The drawing under review shows one solid part. Ordinate dimensions are in mm from its lowest x, y, z. Coordinates: 2 decimals unless noted, no trailing zeros. Order: outer loops, then holes, each group sorted by start corner. A loop starts at its lowest first (then second) coordinate and runs counter-clockwise, first axis right, second up. Notation, with made-up numbers: (3.25, 6) - (51.25, 6) arc R9 ccw to (51.25, 21) - close; hole circle Ø6 at (-39.75, 51). An arc over 180 degrees is marked (long way). Answer in a Markdown table with one row per item.
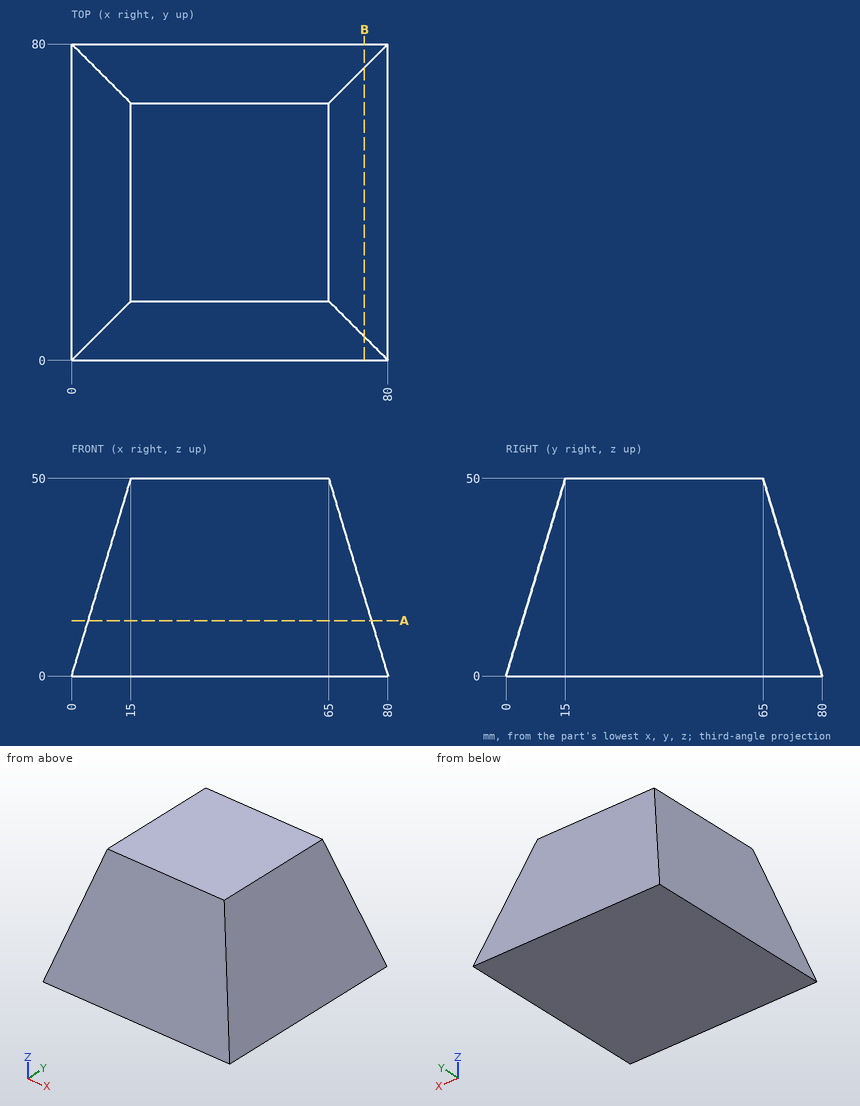
Item 1: We need section A-A, the plane z = 14. Write out the cut boundary in (x, y).
Check values:
| item | result |
|---|---|
| outline | (4.2, 4.2) - (75.8, 4.2) - (75.8, 75.8) - (4.2, 75.8) - close |
Item 2: To check wall thickness, follow line 1 (X direction, y = 59, z = 7); line 2 (Y direction, x = 32.5, z = 28.5); line 3 (Y direction, x = 37.5, z = 29). State the ranges of each line that lie inside material, in increasing order. Write a range as from..to.
Check values:
| item | result |
|---|---|
| line 1 | 2.1..77.9 |
| line 2 | 8.55..71.45 |
| line 3 | 8.7..71.3 |
Item 3: We need section B-B, the plane x = 74. Write out the cut boundary in (y, z).
Check values:
| item | result |
|---|---|
| outline | (0, 0) - (80, 0) - (74, 20) - (6, 20) - close |
Item 4: Clearance check with flat-ended pins moving along their axes: pin 1 Ø2 at (y, z) = (30.5, 14.5) entering from -X; pin 2 Ø8 at (y, z) = (70, 20.5) entering from +X; pin 3 Ø8 at (y, z) = (19.5, 28) entering from -X; pin 4 Ø1 at (x, z) = (8.5, 34.5) entering from -Y. State where each tip first meets the part, or that it passes through.
Check values:
| item | result |
|---|---|
| pin 1 | x = 4.05 |
| pin 2 | x = 75.05 |
| pin 3 | x = 7.2 |
| pin 4 | through |
